For this review, use the dimensioned drawing (mm, ordinates from the lowest corner) and the shaded views. Give positions to 0.01 mm unless a question says otherwise; leave off trailing zeros. Write each loop counter-clockwise with the first axis right and the second up, starting at its lowest first coordinate (ties: lowest second). Pieces come first, ordered by that corner, then holes. Notation, with made-up numbers: M 52.5,-8 L 82.5,-8 A25 ccw 82.5,13 Z; hole C 67.5,42 d2. An arc over 180 degrees is marked long. One line per item, written item: value. Start each with the question number.
Item 1: Consider section B-B, the plane x = 2.54. Write out the cut boundary in (y, z).
Item 2: Consider section A-A, the plane z = 2.54. Write out the cut boundary in (x, y), and give its area (3 significant figures).
Item 3: To check wall thickness, follow probe 1 along X at (y, z) = (0.75, 2.54); probe 2 along Z at (x, y) = (2.54, 0.9); probe 3 along X at (y, z) = (0.65, 1.75). State the ranges of each line that lie inside material, in increasing order.
Item 4: Clearance check with flat-ended pins moving along their axes: pin 1 Ø1.6 at (x, z) = (2.54, 2.54) entering from +Y; pin 2 Ø12 at (x, z) = (12.5, 5) entering from -Y. State where each tip first meets the part, or that it passes through.
Item 5: Consider section C-C, the plane x = 20. Write out the cut boundary in (y, z), and give its area (3 significant figures).
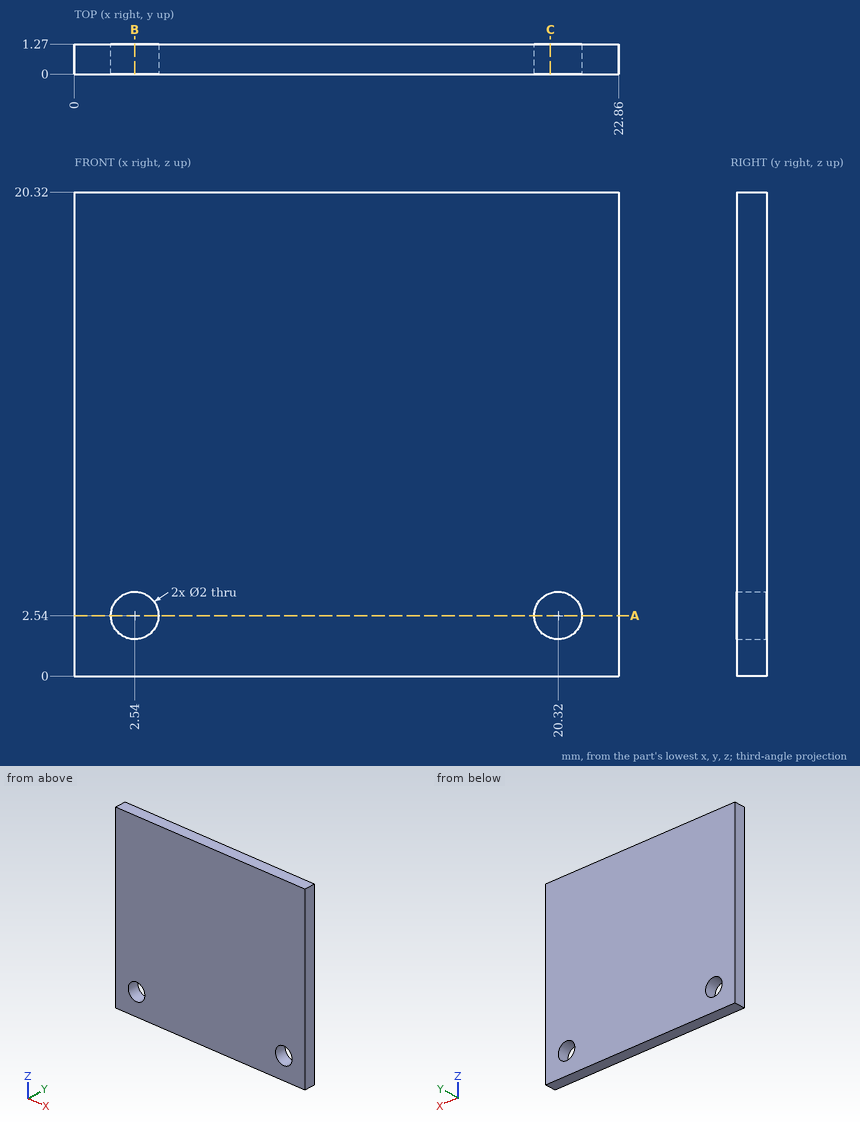
Model answer:
1. outline: M 0,0 L 1.27,0 L 1.27,1.54 L 0,1.54 Z; M 0,3.54 L 1.27,3.54 L 1.27,20.32 L 0,20.32 Z
2. outline: M 0,0 L 1.54,0 L 1.54,1.27 L 0,1.27 Z; M 3.54,0 L 19.32,0 L 19.32,1.27 L 3.54,1.27 Z; M 21.32,0 L 22.86,0 L 22.86,1.27 L 21.32,1.27 Z
2. area: 24.0 mm2
3. probe 1: x = 0 to 1.54, 3.54 to 19.32, 21.32 to 22.86
3. probe 2: z = 0 to 1.54, 3.54 to 20.32
3. probe 3: x = 0 to 1.93, 3.15 to 19.71, 20.93 to 22.86
4. pin 1: passes through
4. pin 2: stops at y = 0
5. outline: M 0,0 L 1.27,0 L 1.27,1.59 L 0,1.59 Z; M 0,3.49 L 1.27,3.49 L 1.27,20.32 L 0,20.32 Z
5. area: 23.4 mm2
